from build123d import *

# Parameters (mm, degrees)
SKETCH_1_R      = 1
SKETCH_1_W      = 67
SKETCH_1_H      = 92
EXTRUDE_1_DEPTH = 1.5
EXTRUDE_2_DEPTH = 1.6
FILLET_1_R      = 0.3
FILLET_2_R      = 0.5


with BuildPart() as part:
    # Эскиз1 → Бобышка-Вытянуть1 (new body)
    with BuildSketch(Plane(origin=(0, 0, 0), x_dir=(1, 0, 0), z_dir=(0, 1, 0))):
        with BuildLine():
            Line((36.75, 49.25), (5.5, 49.25))
            Line((5.5, 49.25), (3, 52.25))
            ThreePointArc((3, 52.25), (0, 55.25), (-3, 52.25))
            Line((-3, 52.25), (-5.300530524, 49.25))
            Line((-5.300530524, 49.25), (-36.75, 49.25))
            Line((-36.75, 49.25), (-36.75, -49.25))
            Line((-36.75, -49.25), (36.75, -49.25))
            Line((36.75, -49.25), (36.75, 49.25))
        make_face()
        with Locations(Location((0, 52.25, 0), (0, 0, 270))):
            Circle(SKETCH_1_R, mode=Mode.SUBTRACT)
        Rectangle(SKETCH_1_W, SKETCH_1_H, mode=Mode.SUBTRACT)
    extrude(amount=EXTRUDE_1_DEPTH)

    # Эскиз2 → Бобышка-Вытянуть2 (add)
    with BuildSketch(Plane(origin=(0, 1.5, 0), x_dir=(1, 0, 0), z_dir=(0, 1, 0))):
        Polygon((35.25, 47.75), (36.75, 49.25), (36.75, -49.25), (-36.75, -49.25), (-36.75, 49.25), (-35.25, 47.75), (-35.25, -47.75), (35.25, -47.75), align=None)
    extrude(amount=EXTRUDE_2_DEPTH)

    # Скругление1
    fillet_1_edges = [part.edges().sort_by_distance(p)[0] for p in [
        (21.125, 0, -49.25),
        (36.75, 0, 0),
        (0, 0, 49.25),
        (-36.75, 0, 0),
        (-21.025265262, 0, -49.25),
        (-4.150265262, 0, -50.75),
        (0, 0, -55.25),
        (4.25, 0, -50.75),
    ]]
    fillet(fillet_1_edges, radius=FILLET_1_R)

    # Скругление2
    fillet_2_edges = [part.edges().sort_by_distance(p)[0] for p in [
        (0, 0, -53.25),
    ]]
    fillet(fillet_2_edges, radius=FILLET_2_R)


solid = part.part
Part model, mm, in its own coordinate system. Coordinates: 2 decimals unless noted, no trailing zeros. Loops run counter-clockwise (first coordinate to the right, second up) from the corner with the lowest first, then second, coordinate; pieces in that order, holes last. Notation, with made-up numbers: M 87.25,-16.5 L 99.25,-16.5 A18 ccw 99.25,7.5 Z; hole C 38,2 d11. An arc over 180 degrees is marked long. Use a Markdown table: item, result. Add a question column.
Q1. Pin check, flat tips, straight feed: P1, Ø1.5, axis at x = -1.5, y = 2.5, coming from the -Z side; P2, Ø1.5, axis at x = -17.5, y = 2, coming from the -Z side. Stop position of each tip, or through.
Q2. Mould opens along Z. For faces 1 (the flat face through (35, 1.5, -8)), 2 (the cylindrical face through (0.3, 0.993, -51.296)), 3 (the cylindrical face through (-4.11, 0.09, -50.66)), 4 (the flat face through (1, 2, 49.25)) say: +Z half, -Z half, draft (parallel to the pull), parting line (faces both ways), or undercut.
Q3. Cut at B-B (z = 10). Write the cut outline in (x, y).
Q4. Probe L1, parallel to X at y = 0.95, z = -52.25; L2, parallel to Z at x = 0.5, y = 1.4; L3, parallel to X at y = 1.65, z = 31.5. List the from-to ranges inside material, lowest first.
Q5. Cut at A-A (x = -13.5). Write the cut outline in (y, z), and give its area (3 significant figures).
Worked out:
| question | item | result |
|---|---|---|
| 1 | P1 | stops at z = 47.75 |
| 1 | P2 | stops at z = -49.25 |
| 2 | face 1 | draft |
| 2 | face 2 | undercut |
| 2 | face 3 | -Z half |
| 2 | face 4 | +Z half |
| 3 | outline | M -36.75,0.3 A0.3 ccw -36.45,0 L -33.5,0 L -33.5,1.5 L -35.25,1.5 L -35.25,3.1 L -36.75,3.1 Z; M 33.5,0 L 36.45,0 A0.3 ccw 36.75,0.3 L 36.75,3.1 L 35.25,3.1 L 35.25,1.5 L 33.5,1.5 Z |
| 4 | L1 | x = -3 to -1, 1 to 3 |
| 4 | L2 | z = -55.21 to -53.12, -51.38 to -46, 46 to 49.25 |
| 4 | L3 | x = -36.75 to -35.25, 35.25 to 36.75 |
| 5 | outline | M 0,-48.95 A0.3 ccw 0.3,-49.25 L 1.5,-49.25 L 1.5,-46 L 0,-46 Z; M 0,46 L 1.5,46 L 1.5,47.75 L 3.1,47.75 L 3.1,49.25 L 0.3,49.25 A0.3 ccw 0,48.95 Z |
| 5 | area | 12.1 mm2 |
